Geometry check sheet. Reference: the model listing, model coordinates, mm. A direction names the side the tool comes from. Coordinates: 2 decimals unless noted, no trailing zeros. Loops run counter-clockwise (first coordinate to the right, second up) from the corner with the lowest first, then second, coordinate; pieces in that order, holes last. Notation, with made-up numbers: M 31,-14.5 L 66,-14.5 A17 ccw 66,0.5 Z; hole C 11,67.5 d8. An arc over 180 degrees is marked long. Use CSV: the item, a comma, the result in double quotes.
```python
from build123d import *

# Parameters (mm, degrees)
SKETCH1_W               = 48.1584
SKETCH1_H               = 36.068
SKETCH1_R               = 8.255
BASE_FLANGE1_DEPTH      = 1.27
EDGE_FLANGE1_DEPTH      = 48.1584
EDGE_FLANGE1_START      = 1.27
EDGE_FLANGE1_PROFILE_W  = 48.1584
EDGE_FLANGE1_PROFILE_H  = 43.2562
EDGE_FLANGE1_PROFILE_R  = 4.73075
EDGE_FLANGE1_FLAT_DEPTH = 1.27
CUT_EXTRUDE7_DEPTH      = 66.234563408
FILLET2_R               = 7.62


# Sheet-metal steps are written as plain solids
with BuildPart() as part:
    # Sketch1 → Base-Flange1 (new body)
    with BuildSketch(Plane(origin=(0, 0, 0), x_dir=(1, 0, 0), z_dir=(0, 1, 0))):
        Rectangle(SKETCH1_W, SKETCH1_H)
        with Locations(Location((0, 0, 0), (0, 0, 270))):
            Circle(SKETCH1_R, mode=Mode.SUBTRACT)
    extrude(amount=-BASE_FLANGE1_DEPTH)

    # Edge-Flange1 bend section (across the edge) → Edge-Flange1 (add)
    with BuildSketch(Plane(origin=(24.0792, 0, -19.304), x_dir=(0, 0, 1), z_dir=(-1, 0, 0))):
        with BuildLine():
            Line((-1.27, 1.27), (0, 1.27))
            ThreePointArc((0, 1.27), (0.371974388, 0.371974388), (1.27, 0))
            Line((1.27, 0), (1.27, -1.27))
            ThreePointArc((1.27, -1.27), (-0.526051224, -0.526051224), (-1.27, 1.27))
        make_face()
    edge_flange1 = extrude(amount=EDGE_FLANGE1_DEPTH)

    # Edge-Flange1 profile (on flange) → Edge-Flange1 flat (add)
    with BuildSketch(Plane(origin=(0, 0, -19.304), x_dir=(-1, 0, 0), z_dir=(0, 0, -1)).offset(EDGE_FLANGE1_START)):
        with Locations((0, 22.8981)):
            Rectangle(EDGE_FLANGE1_PROFILE_W, EDGE_FLANGE1_PROFILE_H)
        with Locations((15.113, 35.56)):
            Circle(EDGE_FLANGE1_PROFILE_R, mode=Mode.SUBTRACT)
        with Locations((-15.113, 35.56)):
            Circle(EDGE_FLANGE1_PROFILE_R, mode=Mode.SUBTRACT)
    edge_flange1_flat = extrude(amount=-EDGE_FLANGE1_FLAT_DEPTH)

    # Mirror1: Edge-Flange1, Edge-Flange1 flat across plane
    add(edge_flange1.mirror(Plane.XY))
    add(edge_flange1_flat.mirror(Plane.XY))

    # Sketch11 → Cut-Extrude7 (cut, through all)
    with BuildSketch(Plane(origin=(0, 0, -20.574), x_dir=(-1, 0, 0), z_dir=(0, 0, -1))):
        with BuildLine():
            Line((24.0792, 35.56), (24.0792, 44.5262))
            Line((24.0792, 44.5262), (-24.0792, 44.5262))
            Line((-24.0792, 44.5262), (-24.0792, 35.56))
            Line((-24.0792, 35.56), (-24.066339002, 35.56))
            ThreePointArc((-24.066339002, 35.56), (-21.115218051, 41.097297222), (-15.113, 42.926))
            ThreePointArc((-15.113, 42.926), (-9.90445145, 40.76854855), (-7.747, 35.56))
            Line((-7.747, 35.56), (7.747, 35.56))
            ThreePointArc((7.747, 35.56), (9.90445145, 40.76854855), (15.113, 42.926))
            ThreePointArc((15.113, 42.926), (21.115218051, 41.097297222), (24.066339002, 35.56))
            Line((24.066339002, 35.56), (24.0792, 35.56))
        make_face()
    extrude(amount=-CUT_EXTRUDE7_DEPTH, mode=Mode.SUBTRACT)

    # Fillet2
    fillet2_edges = [part.edges().sort_by_distance(p)[0] for p in [
        (-7.747, 35.56, -19.939),
        (7.747, 35.56, -19.939),
        (-7.747, 35.56, 19.939),
        (7.747, 35.56, 19.939),
    ]]
    fillet(fillet2_edges, radius=FILLET2_R)


solid = part.part
```
1. Set-up check for faces 4 (the flat face through (0, 22, -19.304)), 5 (the flat face through (-6, -1.27, -8)), 6 (the flat face through (0, 35.56, -20)): record each of +Z, -Z, +X, -X, +Y, -Y from which the full face is reachable in a straight line by a thin tool's end or side.
The answers:
face 4,"+X, -X, +Y"
face 5,"+Z, -Z, +X, -X, -Y"
face 6,"+Z, -Z, +Y"
2. Release check for a two-part mould opening along Y. For faces 1 (the cylindrical face through (16.139, 30.942, 19.948)), 2 (the flat face through (0, 35.56, 20)), 3 (the flat face through (0, 22, 19.304)) record: +Y half, -Y half, draft (parallel to the pull), parting line (faces both ways), or undercut.
The answers:
face 1,"undercut"
face 2,"+Y half"
face 3,"draft"
3. Gauge pin test, flat ends, axial feed: P1, Ø4, axis at x = 9.5, z = -10.5, coming from the +Y side; P2, Ø0.6, axis at x = 1, z = 20.5, coming from the +Y side. Record the tip position at first contact, or that the pin passes through.
The answers:
P1,"y = 0"
P2,"y = 35.56"
4. Section check D-D, the plane y = 33.5. Record the cut outline in (x, z), plus the area to 3 significant figures.
The answers:
outline,"M -24.08,-20.57 L -19.37,-20.57 L -19.37,-19.3 L -24.08,-19.3 Z; M -24.08,19.3 L -19.37,19.3 L -19.37,20.57 L -24.08,20.57 Z; M -10.85,-20.57 L 10.85,-20.57 L 10.85,-19.3 L -10.85,-19.3 Z; M -10.85,19.3 L 10.85,19.3 L 10.85,20.57 L -10.85,20.57 Z; M 19.37,-20.57 L 24.08,-20.57 L 24.08,-19.3 L 19.37,-19.3 Z; M 19.37,19.3 L 24.08,19.3 L 24.08,20.57 L 19.37,20.57 Z"
area,"79.1 mm^2"
5. Section check C-C, the plane y = 6. Record the cut outline in (x, z).
The answers:
outline,"M -24.08,-20.57 L 24.08,-20.57 L 24.08,-19.3 L -24.08,-19.3 Z; M -24.08,19.3 L 24.08,19.3 L 24.08,20.57 L -24.08,20.57 Z"
6. Section check A-A, the plane z = 0. Record the cut outline in (x, y) (3 decimals), plus the area to 3 significant figures.
The answers:
outline,"M -24.079,-1.27 L -8.255,-1.27 L -8.255,0 L -24.079,0 Z; M 8.255,-1.27 L 24.079,-1.27 L 24.079,0 L 8.255,0 Z"
area,"40.2 mm^2"
7. Thickness scan on line 1 (Z direction, x = -17, y = 2.5); line 2 (Y direction, x = 11, z = 7.5); line 3 (X direction, y = -0.95, z = 0) (3 decimals). Record the ranges inside material, lowest first. Write a range as [from, to].
The answers:
line 1,"[-20.57, -19.3], [19.3, 20.57]"
line 2,"[-1.27, 0]"
line 3,"[-24.079, -8.255], [8.255, 24.079]"
8. Section check B-B, the plane x = 0. Record the cut outline in (y, z) (3 decimals).
The answers:
outline,"M -1.27,-18.034 A2.54 ccw 1.27,-20.574 L 35.56,-20.574 L 35.56,-19.304 L 1.27,-19.304 A1.27 cw 0,-18.034 L 0,-8.255 L -1.27,-8.255 Z; M -1.27,8.255 L 0,8.255 L 0,18.034 A1.27 cw 1.27,19.304 L 35.56,19.304 L 35.56,20.574 L 1.27,20.574 A2.54 ccw -1.27,18.034 Z"
